The listing builds one solid part. Answer for the finished solid, in the listing's coordinates (mm). Face numbers are marked on the shaded views. A direction names the side the tool comes from. Give positions to 0.01 mm unless a question says otherwise; leave off trailing zeros. Order: outer loops, then holes, each group sorted by start corner. A loop starts at its lowest first (then second) coordinate and runs counter-clockwise, first axis right, second up.
```python
from build123d import *

# Parameters (mm, degrees)
SKETCH1_R           = 11
BOSS_EXTRUDE1_DEPTH = 1.5
SKETCH2_R           = 9
BOSS_EXTRUDE2_DEPTH = 16.5
BOSS_EXTRUDE3_START = 18
SKETCH1_2_R         = 11
BOSS_EXTRUDE3_DEPTH = 1.5
SKETCH3_R           = 7.5
BOSS_EXTRUDE4_DEPTH = 8
SKETCH4_R           = 3
CUT_EXTRUDE1_DEPTH  = 28.5


with BuildPart() as part:
    # Sketch1 → Boss-Extrude1 (new body)
    with BuildSketch(Plane(origin=(0, 0, 0), x_dir=(1, 0, 0), z_dir=(0, 1, 0))):
        Circle(SKETCH1_R)
    extrude(amount=BOSS_EXTRUDE1_DEPTH)

    # Sketch2 → Boss-Extrude2 (add)
    with BuildSketch(Plane(origin=(0, 1.5, 0), x_dir=(1, 0, 0), z_dir=(0, 1, 0))):
        Circle(SKETCH2_R)
    extrude(amount=BOSS_EXTRUDE2_DEPTH)

    # Sketch1<2> → Boss-Extrude3 (add)
    with BuildSketch(Plane(origin=(0, 0, 0), x_dir=(1, 0, 0), z_dir=(0, 1, 0)).offset(BOSS_EXTRUDE3_START)):
        Circle(SKETCH1_2_R)
    extrude(amount=BOSS_EXTRUDE3_DEPTH)

    # Sketch3 → Boss-Extrude4 (add)
    with BuildSketch(Plane(origin=(0, 19.5, 0), x_dir=(1, 0, 0), z_dir=(0, 1, 0))):
        Circle(SKETCH3_R)
    extrude(amount=BOSS_EXTRUDE4_DEPTH)

    # Sketch4 → Cut-Extrude1 (cut, through all)
    with BuildSketch(Plane.XZ):
        Circle(SKETCH4_R)
    extrude(amount=-CUT_EXTRUDE1_DEPTH, mode=Mode.SUBTRACT)


solid = part.part
```
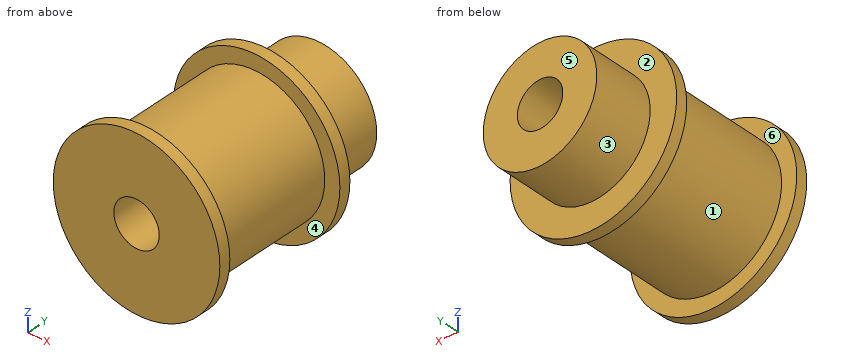
1) Straight lines are drawn through the part: probe 1 along Z at (x, y) = (0, 17.5); probe 2 along Z at (x, y) = (-1, 16); probe 3 along Y at (x, z) = (6, 7.25). For each, find the intervals that lie inside material, in ascending order.
Geometry says:
probe 1: z = -9 to -3, 3 to 9
probe 2: z = -8.94 to -2.83, 2.83 to 8.94
probe 3: y = 0 to 1.5, 18 to 19.5
2) Find section B-B (z = 0). Write down the section's boundary in (x, y), then the cut area to 3 significant figures.
Geometry says:
outline: (-11, 0) - (-3, 0) - (-3, 27.5) - (-7.5, 27.5) - (-7.5, 19.5) - (-11, 19.5) - (-11, 18) - (-9, 18) - (-9, 1.5) - (-11, 1.5) - close; (3, 0) - (11, 0) - (11, 1.5) - (9, 1.5) - (9, 18) - (11, 18) - (11, 19.5) - (7.5, 19.5) - (7.5, 27.5) - (3, 27.5) - close
area: 318 mm2
3) A tool of negligible diameter and unlimited length cuts with its end or side. For the marked faces 5 and 6, from which of +Z, -Z, +X, -X, +Y, -Y can it reach the whole face along a straight path? Write none if from no direction.
Geometry says:
face 5: +Z, -Z, +X, -X, +Y
face 6: none
4) Find section C-C (y = 21.5). Write down the section's boundary in (x, z), then the cut area to 3 significant figures.
Geometry says:
outline: circle Ø15 at (0, 0); hole circle Ø6 at (0, 0)
area: 148 mm2
5) Find section D-D (z = 6). Write down the section's boundary in (x, y).
Geometry says:
outline: (-9.22, 0) - (9.22, 0) - (9.22, 1.5) - (6.71, 1.5) - (6.71, 18) - (9.22, 18) - (9.22, 19.5) - (4.5, 19.5) - (4.5, 27.5) - (-4.5, 27.5) - (-4.5, 19.5) - (-9.22, 19.5) - (-9.22, 18) - (-6.71, 18) - (-6.71, 1.5) - (-9.22, 1.5) - close
6) For a pull along Y with two mould halves and no side action, classify the marked faces 1, 2, 3 and 4 as +Y half, -Y half, draft (parallel to the pull), parting line (faces both ways), or undercut.
Geometry says:
face 1: undercut
face 2: +Y half
face 3: draft
face 4: undercut
7) Find section A-A (x = 0). Write down the section's boundary in (y, z).
Geometry says:
outline: (0, -11) - (1.5, -11) - (1.5, -9) - (18, -9) - (18, -11) - (19.5, -11) - (19.5, -7.5) - (27.5, -7.5) - (27.5, -3) - (0, -3) - close; (0, 3) - (27.5, 3) - (27.5, 7.5) - (19.5, 7.5) - (19.5, 11) - (18, 11) - (18, 9) - (1.5, 9) - (1.5, 11) - (0, 11) - close
8) Given P1, Ø2, axis at x = 6.5, y = 16, coming from the -Z side; P2, Ø8, axis at x = 4, y = 8.5, coming from the +Z side; P3, Ø4, axis at y = 10, z = 2.5, coming from the -X side, each flat-ended and moving along its own axis, determine where each tip first touches the part or whether it passes through.
Geometry says:
P1: stops at z = -7.12
P2: stops at z = 9
P3: stops at x = -8.99
